Geometry check sheet. Reference: the model listing, model coordinates, mm. Coordinates: 2 decimals unless noted, no trailing zeros. Loops run counter-clockwise (first coordinate to the right, second up) from the corner with the lowest first, then second, coordinate; pieces in that order, holes last. Notation, with made-up numbers: (-21, 73) - (-7, 73) arc R24 ccw to (-7, 92) - close; hole circle Ø6 at (63, 61). An arc over 180 degrees is marked (long way). Write item = value, one per line. Start each with the question number.
from build123d import *

# Parameters (mm, degrees)
SKETCH2_R           = 3
SKETCH2_R_2         = 2
BOSS_EXTRUDE1_DEPTH = 40


with BuildPart() as part:
    # Sketch2 → Boss-Extrude1 (new body)
    # profile 1 of 7: a face of its own
    with BuildSketch(Plane.XY):
        Circle(SKETCH2_R)
        Circle(SKETCH2_R_2, mode=Mode.SUBTRACT)
    # profile 2 of 7: a face of its own
    with BuildSketch(Plane.XY):
        with BuildLine():
            Line((0.00424563, 2.999996996), (-1.7278037, 3.002448064))
            Line((-1.7278037, 3.002448064), (-2.595950792, 1.503675326))
            ThreePointArc((-2.595950792, 1.503675326), (-1.496321672, 2.600196426), (0.00424563, 2.999996996))
        make_face()
    # profile 3 of 7: a face of its own
    with BuildSketch(Plane.XY):
        with BuildLine():
            Line((1.736294447, 2.997545929), (0.00424563, 2.999996996))
            ThreePointArc((0.00424563, 2.999996996), (1.503675324, 2.595950793), (2.600196428, 1.496321669))
            Line((2.600196428, 1.496321669), (1.736294447, 2.997545929))
        make_face()
    # profile 4 of 7: a face of its own
    with BuildSketch(Plane.XY):
        with BuildLine():
            Line((3.464098147, -0.004902135), (2.600196428, 1.496321669))
            ThreePointArc((2.600196428, 1.496321669), (2.898326179, 0.774406456), (3, 0))
            ThreePointArc((3, 0), (2.897227326, -0.778507431), (2.595950787, -1.503675335))
            Line((2.595950787, -1.503675335), (3.464098147, -0.004902135))
        make_face()
    # profile 5 of 7: a face of its own
    with BuildSketch(Plane.XY):
        with BuildLine():
            ThreePointArc((2.595950787, -1.503675335), (1.496321666, -2.60019643), (-0.004245634, -2.999996996))
            Line((-0.004245634, -2.999996996), (1.7278037, -3.002448064))
            Line((1.7278037, -3.002448064), (2.595950787, -1.503675335))
        make_face()
    # profile 6 of 7: a face of its own
    with BuildSketch(Plane.XY):
        with BuildLine():
            ThreePointArc((-0.004245634, -2.999996996), (-1.503675323, -2.595950794), (-2.600196425, -1.496321674))
            Line((-2.600196425, -1.496321674), (-1.736294447, -2.997545929))
            Line((-1.736294447, -2.997545929), (-0.004245634, -2.999996996))
        make_face()
    # profile 7 of 7: a face of its own
    with BuildSketch(Plane.XY):
        with BuildLine():
            ThreePointArc((-2.600196425, -1.496321674), (-2.999996996, 0.004245633), (-2.595950792, 1.503675326))
            Line((-2.595950792, 1.503675326), (-3.464098147, 0.004902135))
            Line((-3.464098147, 0.004902135), (-2.600196425, -1.496321674))
        make_face()
    extrude(amount=BOSS_EXTRUDE1_DEPTH)


solid = part.part
(1) Draft check along X on faces 1 (the face through (0, -2, 20)), 2 (the face through (1, 2, 0)). Enter one of: pulls with the +X half, pulls with the -X half, needs draft (parallel to the pull), parting line crosses it, or undercut.
(2) Sectioned sample at A-A on z = 9.5. Enter the section's corners in (x, y), plus the area to 3 significant figures.
(3) Depth check by flat-ended pin: pin 1 (1 mm diameter, centred on x = -2.5, z = 35, fed in from -Y). Enter the tip coordinate at first touch or a pass-through.
(4) Sectioned sample at D-D on y = -2.5. Enter the section's corners in (x, z).
(5) Scan lines: line 1 (Y direction, x = 0, z = 8); line 2 (Y direction, x = -1.75, z = 30); line 3 (X direction, y = -1.25, z = 23). Record each from-to range of solid material in increasing order.
(6) Sectioned sample at C-C on y = 0.5. Enter the section's corners in (x, z).
(7) Sectioned sample at B-B on x = -0.5. Enter the section's corners in (y, z).
Working result:
q1.face_1 = undercut
q1.face_2 = needs draft
q2.outline = (-3.46, 0) - (-1.74, -3) - (1.73, -3) - (3.46, 0) - (1.74, 3) - (-1.73, 3) - close; hole circle Ø4 at (0, 0)
q2.area = 18.6 mm2
q3.pin_1 = -2.54
q4.outline = (-2.02, 0) - (2.02, 0) - (2.02, 40) - (-2.02, 40) - close
q5.line_1 = -3 to -2, 2 to 3
q5.line_2 = -2.97 to -0.97, 0.97 to 2.96
q5.line_3 = -2.74 to -1.56, 1.56 to 2.74
q6.outline = (-3.18, 0) - (-1.94, 0) - (-1.94, 40) - (-3.18, 40) - close; (1.94, 0) - (3.17, 0) - (3.17, 40) - (1.94, 40) - close
q7.outline = (-3, 0) - (-1.94, 0) - (-1.94, 40) - (-3, 40) - close; (1.94, 0) - (3, 0) - (3, 40) - (1.94, 40) - close
